The listing builds one solid part. Answer for the finished solid, in the listing's coordinates (mm). A direction names the side the tool comes from. Give positions to 0.01 mm unless a question says otherwise; leave off trailing zeros. Loops run counter-clockwise (first coordinate to the right, second up) from the corner with the lowest first, then second, coordinate; pieces in that order, holes last.
Item 1: Each of these flat-tipped pins is pushed along its axis until it touches: pin 1 Ø7.5 at (x, z) = (44.45, 0) entering from -Y; pin 2 Ø1 at (y, z) = (-1, -7) entering from +X; pin 3 Ø0.6 at (y, z) = (-2, -3) entering from +X; pin 4 Ø10 at (x, y) = (14.5, -13) entering from -Z. Where does it stop, or does it pass through?
Item 2: The mould has two halves that part along X. Classify faces 1 (the face through (-38.513, -22.194, 5.34)), 2 (the face through (28.43, 0.04, -0.95)), 3 (the face through (22.6, -2.54, -2.3)), 4 (the face through (3.477, -12.215, -0.133)): pulls with the +X half, pulls with the -X half, needs draft (parallel to the pull), parting line crosses it, or undercut.
Item 3: Section D-D, the plane z = 8 is taken. Give the vertices of the cut face in (x, y) (3 decimals), and give its area (3 significant figures).
Item 4: Section A-A, the plane x = 25.4 is taken. Give the vertices of the cut face in (y, z) (3 decimals), and give its area (3 significant figures).
Item 5: Section B-B, the plane z = -4 is taken. Give the vertices of the cut face in (x, y) (3 decimals), and give its area (3 significant figures).
Item 6: Section C-C, the plane y = 4 is taken. Give the vertices of the cut face in (x, z) (3 decimals), and give its area (3 significant figures).
Item 7: Consider line 1 along X through (y, z) = (0.6, 0) (3 decimals); line 2 along Z through (x, y) = (25.4, 1) (3 decimals); line 3 along X through (y, z) = (2, -1.5). Determine where each line is inside the solid, lowest interval first.
Item 8: A tool of negligible diameter and unlimited length cuts with its end or side. For faces 5 (the face through (48, -1.27, 0)), 6 (the face through (48, 1.27, 0)), 7 (the face through (-35, -20, 1.27)), 8 (the face through (-20.48, -14.757, -0.133)), from which of +Z, -Z, +X, -X, +Y, -Y can it reach the whole face along a straight path? Write none if from no direction.
Autodesk Inventor part; units mm, degrees
ref_plane "YZ Plane" through (0, 0, 0) normal (1, 0, 0) x (0, 1, 0)
ref_plane "XZ Plane" through (0, 0, 0) normal (0, 1, 0) x (-1, 0, 0)
ref_plane "XY Plane" through (0, 0, 0) normal (0, 0, 1) x (1, 0, 0)
sketch "Sketch1" plane through (0, 0, 0) normal (0, 0, 1) x (1, 0, 0)
  circle A0 centre (0, 0) radius 9.525
  line L0 (38.1, 1.27) -> (38.1, 2.54)
  line L1 (38.1, -1.27) -> (38.1, -2.54)
  line L2 (38.1, -2.54) -> (12.4434, -2.54)
  line L3 (38.1, 2.54) -> (12.4434, 2.54)
  line L4 (38.1, 0) -> (44.45, 0)
  line L5 (44.45, 0) -> (44.45, 1.27)
  line L6 (44.45, 1.27) -> (38.1, 1.27)
  line L7 (44.45, -1.27) -> (44.45, 0)
  line L8 (44.45, -1.27) -> (38.1, -1.27)
  line L9 (-38.4948, -22.225) -> (-37.2248, -24.4247)
  line L10 (-37.2248, -24.4247) -> (-9.5063, -8.4214)
  line L11 (-38.4948, -22.225) -> (-39.7648, -20.0253)
  line L12 (-39.7648, -20.0253) -> (-12.0463, -4.022)
  arc A1 (12.4434, 2.54) -> (-12.0463, -4.022) centre (0, 0) ccw
  arc A2 (-9.5063, -8.4214) -> (12.4434, -2.54) centre (0, 0) ccw
  dimension "d1" = 19.05
  dimension "d5" = 38.1
  dimension "d6" = 2.54
  dimension "d7" = 2.54
  dimension "d8" = 6.35
  dimension "d9" = 1.27
  dimension "d11" = 44.45
  dimension "d12" = 2.54
  dimension "d13" = 2.54
  dimension "d36" = 12.7
extrude "Extrusion1" add sketch "Sketch1" along normal mid plane 19.05
sketch "Sketch4" plane through (38.1, 1.27, 9.525) normal (0, 1, 0) x (1, 0, 0)
  arc A0 (6.35, 0) -> (6.35, 19.05) centre (6.35, 9.525) ccw
  line L0 (6.35, 19.05) -> (6.35, 0)
  line L1 (0, 0) -> (6.35, 0)
  point P0 (-38.1, 9.525)
  dimension "d16" = 9.525
extrude "Extrusion2" add sketch "Sketch4" against normal blind 2.54
sketch "Sketch5" plane through (38.1, 1.27, 9.525) normal (0, 1, 0) x (1, 0, 0)
  arc A0 (6.35, 0) -> (6.35, 19.05) centre (6.35, 9.525) ccw
  circle A1 centre (6.35, 9.525) radius 3.175
  circle A2 centre (-11.5739, 9.525) radius 3.175
  point P0 (-38.1, 9.525)
  dimension "d19" = 6.35
extrude "Extrusion3" cut sketch "Sketch5" against normal through all contours A1
sketch "Sketch6" plane through (12.4434, 2.54, 9.525) normal (0, 1, 0) x (1, 0, 0)
  circle A0 centre (12.9566, 9.525) radius 3.175
  line L0 (25.6566, 19.05) -> (0, 19.05)
  line L1 (25.6566, 19.05) -> (25.6566, 0)
  point P0 (-12.4434, 9.525)
  dimension "d23" = 6.35
  dimension "d24" = 9.525
  dimension "d25" = 12.7
extrude "Extrusion4" cut sketch "Sketch6" against normal through all
sketch "Sketch7" plane through (-39.7648, -20.0253, 9.525) normal (-0.5, 0.866, 0) x (0.866, 0.5, 0)
  arc A0 (7.7813, 8.255) -> (7.7813, 10.795) centre (12.7, 9.525) ccw
  line L0 (0, 0) -> (0, 19.05)
  line L1 (0, 19.05) -> (32.0066, 19.05)
  line L2 (7.7813, 10.795) -> (0, 10.795)
  line L3 (7.7813, 8.255) -> (0, 8.255)
  line L4 (0, 10.795) -> (0, 8.255)
  point P0 (44.45, 9.525)
  dimension "d28" = 10.16
  dimension "d29" = 12.7
  dimension "d33" = 9.525
extrude "Extrusion5" cut sketch "Sketch7" against normal through all
properties part number "HW 8 Part 4"
Worked answers:
1. pin 1: stops at y = -1.27
1. pin 2: stops at x = 51.41
1. pin 3: stops at x = 38.1
1. pin 4: passes through
2. face 1: pulls with the -X half
2. face 2: undercut
2. face 3: needs draft
2. face 4: undercut
3. outline: (-39.765, -20.025) - (-37.225, -24.425) - (-9.506, -8.421) arc R12.7 ccw to (12.443, -2.54) - (38.1, -2.54) - (38.1, -1.27) - (49.62, -1.27) - (49.62, 1.27) - (38.1, 1.27) - (38.1, 2.54) - (12.443, 2.54) arc R12.7 ccw (long way) to (-12.046, -4.022) - close; hole circle Ø19.05 at (0, 0)
3. area: 542 mm2
4. outline: (-2.54, -9.525) - (2.54, -9.525) - (2.54, -3.175) - (-2.54, -3.175) - close; (-2.54, 3.175) - (2.54, 3.175) - (2.54, 9.525) - (-2.54, 9.525) - close
4. area: 64.5 mm2
5. outline: (-39.765, -20.025) - (-37.225, -24.425) - (-28.938, -19.64) - (-31.478, -15.241) - close; (-26.054, -12.11) - (-23.514, -16.509) - (-9.506, -8.421) arc R12.7 ccw to (12.443, -2.54) - (38.1, -2.54) - (38.1, -1.27) - (53.094, -1.27) - (53.094, 1.27) - (38.1, 1.27) - (38.1, 2.54) - (12.443, 2.54) arc R12.7 ccw (long way) to (-12.046, -4.022) - close; hole circle Ø19.05 at (0, 0)
5. area: 519 mm2
6. outline: (-12.054, -9.525) - (-8.644, -9.525) - (-8.644, 9.525) - (-12.054, 9.525) - close; (8.644, -9.525) - (12.054, -9.525) - (12.054, 9.525) - (8.644, 9.525) - close
6. area: 130 mm2
7. line 1: x = -12.686 to -9.506, 9.506 to 22.225, 28.575 to 41.275, 47.625 to 53.975
7. line 2: z = -9.525 to -3.175, 3.175 to 9.525
7. line 3: x = -12.54 to -9.31, 9.31 to 22.6, 28.2 to 38.1
8. face 5: +Z, -Z, +X, -Y
8. face 6: +Z, -Z, +X, +Y
8. face 7: +X, -X, +Y, -Y
8. face 8: +Z, -Z, -Y
